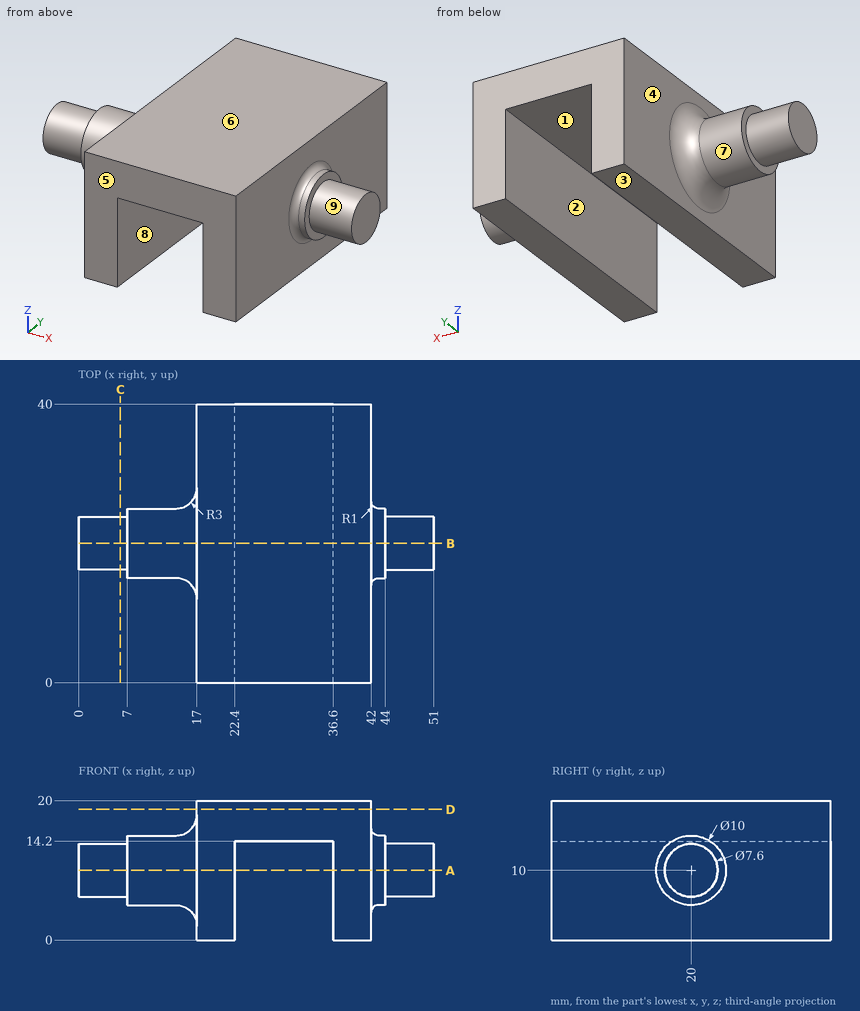
Could you check a few things on this drawing? It's one solid part, dimensions in mm from its lowest x, y, z. A direction names the side the tool comes from. Round coordinates to 2 decimals unless told otherwise and drop trailing zeros. Loops run counter-clockwise (first coordinate to the right, second up) from the corner with the lowest first, then second, coordinate; pieces in that order, holes last. Notation, with made-up numbers: (88.5, 48) -> (142.5, 48) arc R32 ccw to (142.5, 75) -> close; hole circle Ø11 at (34.25, 67). An arc over 180 degrees is marked (long way). Write each question's results on one line, items separated by ' | '.
(1) If we section it at C-C, the plane x = 6: List the corners of the cut face in (y, z) for me.
Worked answers:
outline: circle Ø7.6 at (20, 10)
(2) If I drill on L1, parallel to X at y = 19, z = 11.75; L2, parallel to X at y = 26, z = 1.5; L3, parallel to Z at x = 27, y = 22.5, over which ranges is the centre line in solid material (lowest first)?
Worked answers:
L1: 0 to 22.4, 36.6 to 51 | L2: 17 to 22.4, 36.6 to 42 | L3: 14.2 to 20
(3) For the marked faces 5, 6, 7, 8 and 9, which set-ups out of +Z, -Z, +X, -X, +Y, -Y let a thin tool reach every point of the face, with its end or its side?
Worked answers:
face 5: +Z, -Z, +X, -X, -Y | face 6: +Z, +X, -X, +Y, -Y | face 7: -X | face 8: -Z, +Y, -Y | face 9: +X
(4) We'd pull the mould along X, two halves only. Please class the marked faces 1, 2, 3 and 4: released by +X, released by -X, zero draft, split by the parting line, or undercut.
Worked answers:
face 1: undercut | face 2: undercut | face 3: zero draft | face 4: released by -X
(5) If we section it at B-B, the plane y = 20: List the corners of the cut face in (x, z) for me.
Worked answers:
outline: (0, 6.2) -> (7, 6.2) -> (7, 5) -> (14, 5) arc R3 cw to (17, 2) -> (17, 0) -> (22.4, 0) -> (22.4, 14.2) -> (36.6, 14.2) -> (36.6, 0) -> (42, 0) -> (42, 4) arc R1 cw to (43, 5) -> (44, 5) -> (44, 6.2) -> (51, 6.2) -> (51, 13.8) -> (44, 13.8) -> (44, 15) -> (43, 15) arc R1 cw to (42, 16) -> (42, 20) -> (17, 20) -> (17, 18) arc R3 cw to (14, 15) -> (7, 15) -> (7, 13.8) -> (0, 13.8) -> close
(6) For P1, Ø15.5, axis at x = 32, y = 29, coming from the -Z side; P2, Ø6, axis at y = 11.5, z = 10, coming from the +X side; P3, Ø1, axis at x = 13, y = 24, coming from the +Z side; P4, Ø4.5, axis at y = 29.5, z = 5.5, coming from the +X side, each with a flat end and sliding along its axis, tell me the tip position at first contact or that it passes through.
Worked answers:
P1: z = 0 | P2: x = 42.13 | P3: z = 13.57 | P4: x = 42
(7) If we section it at D-D, the plane z = 18.75: List the corners of the cut face in (x, y) for me.
Worked answers:
outline: (17, 0) -> (42, 0) -> (42, 40) -> (17, 40) -> close
(8) If we section it at A-A, the plane z = 10: List the corners of the cut face in (x, y) for me, then the cut area to 3 significant figures.
Worked answers:
outline: (0, 16.2) -> (7, 16.2) -> (7, 15) -> (14, 15) arc R3 cw to (17, 12) -> (17, 0) -> (22.4, 0) -> (22.4, 40) -> (17, 40) -> (17, 28) arc R3 cw to (14, 25) -> (7, 25) -> (7, 23.8) -> (0, 23.8) -> close; (36.6, 0) -> (42, 0) -> (42, 14) arc R1 cw to (43, 15) -> (44, 15) -> (44, 16.2) -> (51, 16.2) -> (51, 23.8) -> (44, 23.8) -> (44, 25) -> (43, 25) arc R1 cw to (42, 26) -> (42, 40) -> (36.6, 40) -> close | area: 663 mm2
